```python
from build123d import *

# Parameters (mm, degrees)
SKETCH1_W           = 22
SKETCH1_H           = 1.9
BOSS_EXTRUDE1_DEPTH = 31.1
CUT_EXTRUDE2_REACH  = 3.9
CUT_EXTRUDE3_REACH  = 3.9
CUT_EXTRUDE4_DEPTH  = 0.85
CHAMFER1_SIZE       = 0.3
SKETCH2_8_W         = 1.9
SKETCH2_8_H         = 13
CUT_EXTRUDE6_DEPTH  = 1.1
CUT_EXTRUDE7_DEPTH  = 1.15
SKETCH2_10_W        = 1.137
SKETCH2_10_H        = 1.05
CUT_EXTRUDE8_DEPTH  = 0.75
SKETCH2_11_W        = 1.137
SKETCH2_11_H        = 4.7
CUT_EXTRUDE9_DEPTH  = 0.4
CUT_EXTRUDE10_DEPTH = 0.2
CUT_EXTRUDE12_DEPTH = 0.1


with BuildPart() as part:
    # Sketch1 → Boss-Extrude1 (new body)
    with BuildSketch(Plane(origin=(0, 0, 0), x_dir=(1, 0, 0), z_dir=(0, 1, 0))):
        Rectangle(SKETCH1_W, SKETCH1_H)
    extrude(amount=BOSS_EXTRUDE1_DEPTH)

    # Sketch2 → Cut-Extrude2 (cut, up to next)
    with BuildSketch(Plane.XY.offset(0.95), mode=Mode.PRIVATE) as cut_extrude2_sk1:
        with BuildLine():
            Line((-11, 31.1), (-11, 28.2))
            ThreePointArc((-11, 28.2), (0, 30.9), (11, 28.2))
            Line((11, 28.2), (11, 31.1))
            Line((11, 31.1), (-11, 31.1))
        make_face()
    cut_extrude2_tool1 = extrude(cut_extrude2_sk1.sketch, amount=-CUT_EXTRUDE2_REACH, mode=Mode.PRIVATE) & part.part
    add(cut_extrude2_tool1.solids().sort_by_distance((10.778097, 29.65, 0.95))[0], mode=Mode.SUBTRACT)

    # Sketch2_4 → Cut-Extrude3 (cut, up to next)
    with BuildSketch(Plane.XY.offset(0.95), mode=Mode.PRIVATE) as cut_extrude3_sk1:
        Polygon((-11, 26.2), (-11, 22.2), (-10.65, 22.35), (-10.65, 26.05), align=None)
    cut_extrude3_tool1 = extrude(cut_extrude3_sk1.sketch, amount=-CUT_EXTRUDE3_REACH, mode=Mode.PRIVATE) & part.part
    add(cut_extrude3_tool1.solids().sort_by_distance((-10.827273, 24.2, 0.95))[0], mode=Mode.SUBTRACT)
    # Sketch2_4 → Cut-Extrude3 (cut, up to next)
    with BuildSketch(Plane.XY.offset(0.95), mode=Mode.PRIVATE) as cut_extrude3_sk2:
        Polygon((11, 22.2), (11, 26.2), (10.65, 26.05), (10.65, 22.35), align=None)
    cut_extrude3_tool2 = extrude(cut_extrude3_sk2.sketch, amount=-CUT_EXTRUDE3_REACH, mode=Mode.PRIVATE) & part.part
    add(cut_extrude3_tool2.solids().sort_by_distance((10.827273, 24.2, 0.95))[0], mode=Mode.SUBTRACT)
    # Sketch2_4 → Cut-Extrude3 (cut, up to next)
    with BuildSketch(Plane.XY.offset(0.95), mode=Mode.PRIVATE) as cut_extrude3_sk3:
        with BuildLine():
            Line((11, 0), (11, 3))
            ThreePointArc((11, 3), (10.6190025, 2.145891674), (10.1, 1.36788362))
            ThreePointArc((10.1, 1.36788362), (9.365445636, 0.607390694), (8.5, 0))
            Line((8.5, 0), (11, 0))
        make_face()
    cut_extrude3_tool3 = extrude(cut_extrude3_sk3.sketch, amount=-CUT_EXTRUDE3_REACH, mode=Mode.PRIVATE) & part.part
    add(cut_extrude3_tool3.solids().sort_by_distance((10.267991, 0.865194, 0.95))[0], mode=Mode.SUBTRACT)

    # Sketch2_5 → Cut-Extrude4 (cut)
    with BuildSketch(Plane.XY.offset(0.95)):
        with BuildLine():
            Line((11, 10.7), (11, 12.8))
            Line((11, 12.8), (10.25, 12.8))
            ThreePointArc((10.25, 12.8), (9.2, 11.75), (10.25, 10.7))
            Line((10.25, 10.7), (11, 10.7))
        make_face()
    extrude(amount=-CUT_EXTRUDE4_DEPTH, mode=Mode.SUBTRACT)

    # Chamfer1
    chamfer1_edges = [part.edges().sort_by_distance(p)[0] for p in [
        (-1.25, 0, 0.95),
    ]]
    chamfer(chamfer1_edges, length=CHAMFER1_SIZE)

    # Sketch2_8 → Cut-Extrude6 (cut)
    with BuildSketch(Plane.XY.offset(0.95)):
        with Locations((-9.15, 6.5)):
            Rectangle(SKETCH2_8_W, SKETCH2_8_H)
    extrude(amount=-CUT_EXTRUDE6_DEPTH, mode=Mode.SUBTRACT)

    # Sketch2_9 → Cut-Extrude7 (cut)
    with BuildSketch(Plane.XY.offset(0.95)):
        with BuildLine():
            ThreePointArc((8.5, 0), (9.365445636, 0.607390694), (10.1, 1.36788362))
            Line((10.1, 1.36788362), (10.1, 9.3))
            Line((10.1, 9.3), (7.9, 9.3))
            Line((7.9, 9.3), (7.9, 0))
            Line((7.9, 0), (8.5, 0))
        make_face()
    extrude(amount=-CUT_EXTRUDE7_DEPTH, mode=Mode.SUBTRACT)

    # Sketch2_10 → Cut-Extrude8 (cut)
    with BuildSketch(Plane.XY.offset(0.95)):
        with Locations((-6.4315, 0.525)):
            Rectangle(SKETCH2_10_W, SKETCH2_10_H)
        with Locations((-5.0245, 0.525)):
            Rectangle(SKETCH2_10_W, SKETCH2_10_H)
        with Locations((-3.6175, 0.525)):
            Rectangle(SKETCH2_10_W, SKETCH2_10_H)
        with Locations((-2.2105, 0.525)):
            Rectangle(SKETCH2_10_W, SKETCH2_10_H)
        with Locations((-0.8035, 0.525)):
            Rectangle(SKETCH2_10_W, SKETCH2_10_H)
        with Locations((0.6035, 0.525)):
            Rectangle(SKETCH2_10_W, SKETCH2_10_H)
        with Locations((2.0105, 0.525)):
            Rectangle(SKETCH2_10_W, SKETCH2_10_H)
        with Locations((3.4175, 0.525)):
            Rectangle(SKETCH2_10_W, SKETCH2_10_H)
        with Locations((4.8245, 0.525)):
            Rectangle(SKETCH2_10_W, SKETCH2_10_H)
        with Locations((6.2315, 0.525)):
            Rectangle(SKETCH2_10_W, SKETCH2_10_H)
    extrude(amount=-CUT_EXTRUDE8_DEPTH, mode=Mode.SUBTRACT)

    # Sketch2_11 → Cut-Extrude9 (cut)
    with BuildSketch(Plane.XY.offset(0.95)):
        with Locations((-6.4315, 3.4)):
            Rectangle(SKETCH2_11_W, SKETCH2_11_H)
        with Locations((-5.0245, 3.4)):
            Rectangle(SKETCH2_11_W, SKETCH2_11_H)
        with Locations((-3.6175, 3.4)):
            Rectangle(SKETCH2_11_W, SKETCH2_11_H)
        with Locations((-2.2105, 3.4)):
            Rectangle(SKETCH2_11_W, SKETCH2_11_H)
        with Locations((-0.8035, 3.4)):
            Rectangle(SKETCH2_11_W, SKETCH2_11_H)
        with Locations((0.6035, 3.4)):
            Rectangle(SKETCH2_11_W, SKETCH2_11_H)
        with Locations((2.0105, 3.4)):
            Rectangle(SKETCH2_11_W, SKETCH2_11_H)
        with Locations((3.4175, 3.4)):
            Rectangle(SKETCH2_11_W, SKETCH2_11_H)
        with Locations((4.8245, 3.4)):
            Rectangle(SKETCH2_11_W, SKETCH2_11_H)
        with Locations((6.2315, 3.4)):
            Rectangle(SKETCH2_11_W, SKETCH2_11_H)
    extrude(amount=-CUT_EXTRUDE9_DEPTH, mode=Mode.SUBTRACT)

    # Sketch5 → Cut-Extrude10 (cut)
    with BuildSketch(Plane(origin=(0, 0, -0.95), x_dir=(-1, 0, 0), z_dir=(0, 0, -1))):
        with BuildLine():
            Line((-9.4, 4.6), (-9.4, 27.207255635))
            ThreePointArc((-9.4, 27.207255635), (0, 29.3), (9.4, 27.207255635))
            Line((9.4, 27.207255635), (9.4, 4.6))
            Line((9.4, 4.6), (-9.4, 4.6))
        make_face()
    extrude(amount=-CUT_EXTRUDE10_DEPTH, mode=Mode.SUBTRACT)

    # Sketch6 → Cut-Extrude12 (cut)
    with BuildSketch(Plane(origin=(0, 0, -0.95), x_dir=(-1, 0, 0), z_dir=(0, 0, -1))):
        Polygon((-3.15, 3.48074093), (3.15, 3.48074093), (0, 1.58074093), align=None)
    extrude(amount=-CUT_EXTRUDE12_DEPTH, mode=Mode.SUBTRACT)


solid = part.part
```
Work out the finished part from the listing and answer in its coordinate system (mm). A direction names the side the tool comes from. Give positions to 0.01 mm unless a question says otherwise; leave off trailing zeros. Write each loop counter-clockwise with the first axis right and the second up, starting at its lowest first coordinate (ties: lowest second). Pieces come first, ordered by that corner, then holes.
(1) Which of the six approach directions +Z, -Z, +X, -X, +Y, -Y give full straight-line access (tool end or side, diameter ignored) to faces 1 (the flat face through (0, 17, -0.75)), 2 (the flat face through (2, 0.5, 0.2))?
Final values:
face 1: -Z
face 2: +Z, -Y
(2) Straight lines are drawn through the part: line 1 (X direction, y = 4, z = -0.05); line 2 (X direction, y = 9.5, z = 0.6); line 3 (X direction, y = 2, z = -0.1). For each, find the intervals that lie inside material, in ascending order.
Final values:
line 1: x = -11 to -10.1, -8.2 to 7.9, 10.1 to 11
line 2: x = -11 to -10.1, -8.2 to 11
line 3: x = -11 to -10.1, -8.2 to 7.9, 10.1 to 10.54
(3) The part is cut by section C-C on y = 18. Write down the section's boundary in (x, z), plus the area to 3 significant figures.
Final values:
outline: (-11, -0.95) - (-9.4, -0.95) - (-9.4, -0.75) - (9.4, -0.75) - (9.4, -0.95) - (11, -0.95) - (11, 0.95) - (-11, 0.95) - close
area: 38.0 mm2
(4) A flat-ended cylindrical pin translates along its axis: pin 1 Ø0.8 at (y, z) = (2, 0.5) entering from +X. Find the tip coordinate at first contact, or state that the pin passes through.
Final values:
pin 1: stops at x = 10.75
(5) The part is cut by section D-D on x = -2. Write down the section's boundary in (y, z), plus the area to 3 significant figures.
Final values:
outline: (0, -0.95) - (2.79, -0.95) - (2.79, -0.85) - (3.48, -0.85) - (3.48, -0.95) - (4.6, -0.95) - (4.6, -0.75) - (29.21, -0.75) - (29.21, -0.95) - (30.82, -0.95) - (30.82, 0.95) - (5.75, 0.95) - (5.75, 0.55) - (1.05, 0.55) - (1.05, 0.2) - (0, 0.2) - close
area: 50.9 mm2
(6) The part is cut by section B-B on x = 4.75. Write down the section's boundary in (y, z), plus the area to 3 significant figures.
Final values:
outline: (0, -0.95) - (4.6, -0.95) - (4.6, -0.75) - (28.78, -0.75) - (28.78, -0.95) - (30.42, -0.95) - (30.42, 0.95) - (5.75, 0.95) - (5.75, 0.55) - (1.05, 0.55) - (1.05, 0.2) - (0, 0.2) - close
area: 50.3 mm2
(7) The mould has two halves that part along X. Classify faces 3 (the flat face through (-9, 7, -0.15)), 4 (the flat face through (-10, 13, -0.95)), 5 (the cylindrical face through (-0.2, 30.9, 0)): pulls with the +X half, pulls with the -X half, needs draft (parallel to the pull), parting line crosses it, or undercut.
Final values:
face 3: undercut
face 4: needs draft
face 5: parting line crosses it
(8) The part is cut by section A-A on y = 11.75. Write down the section's boundary in (x, z).
Final values:
outline: (-11, -0.95) - (-9.4, -0.95) - (-9.4, -0.75) - (9.4, -0.75) - (9.4, -0.95) - (11, -0.95) - (11, 0.1) - (9.2, 0.1) - (9.2, 0.95) - (-8.2, 0.95) - (-8.2, -0.15) - (-10.1, -0.15) - (-10.1, 0.95) - (-11, 0.95) - close
